Here's the drawing with two shaded views (mm, measured from the low corner). I have some questions. Coordinates: 2 decimals unless noted, no trailing zeros. Order: outer loops, then holes, each group sorted by start corner. A loop starts at its lowest first (then second) coordinate and runs counter-clockwise, first axis right, second up. Notation, with made-up numbers: (45.5, 44.5) - (64.5, 44.5) arc R26 ccw to (64.5, 66.5) - close; hole circle Ø10 at (21.25, 8.25). An arc over 180 degrees is marked (long way). Answer as a JSON object with one key per item and string values. Group by question number.
(1) Will these pins go through, and if not, where does the flat tip stop? P1, Ø1, axis at x = 5.5, z = 15, coming from the +Y side; P2, Ø5, axis at x = 4.5, z = 14.5, coming from the +Y side; P3, Ø6, axis at x = 14, z = 19.5, coming from the +Y side; P4, Ø3, axis at x = 14.5, y = 56.5, coming from the +Z side (1 decimal).
(2) Imagine slicing it at C-C, the plane z = 3. Write out the boundary of the cut face in (x, y).
(3) Please list where these lines run through material, in increasing order: probe 1 along Z at (x, y) = (10.5, 50.8); probe 2 along Y at (x, z) = (6, 13.75); probe 3 along Y at (x, z) = (10, 14.5).
(4) We'd pull the mould along Z, two halves only. Please class the marked faces 1, 2, 3 and 4: pulls with the +Z half, pulls with the -Z half, needs draft (parallel to the pull), parting line crosses it, or undercut.
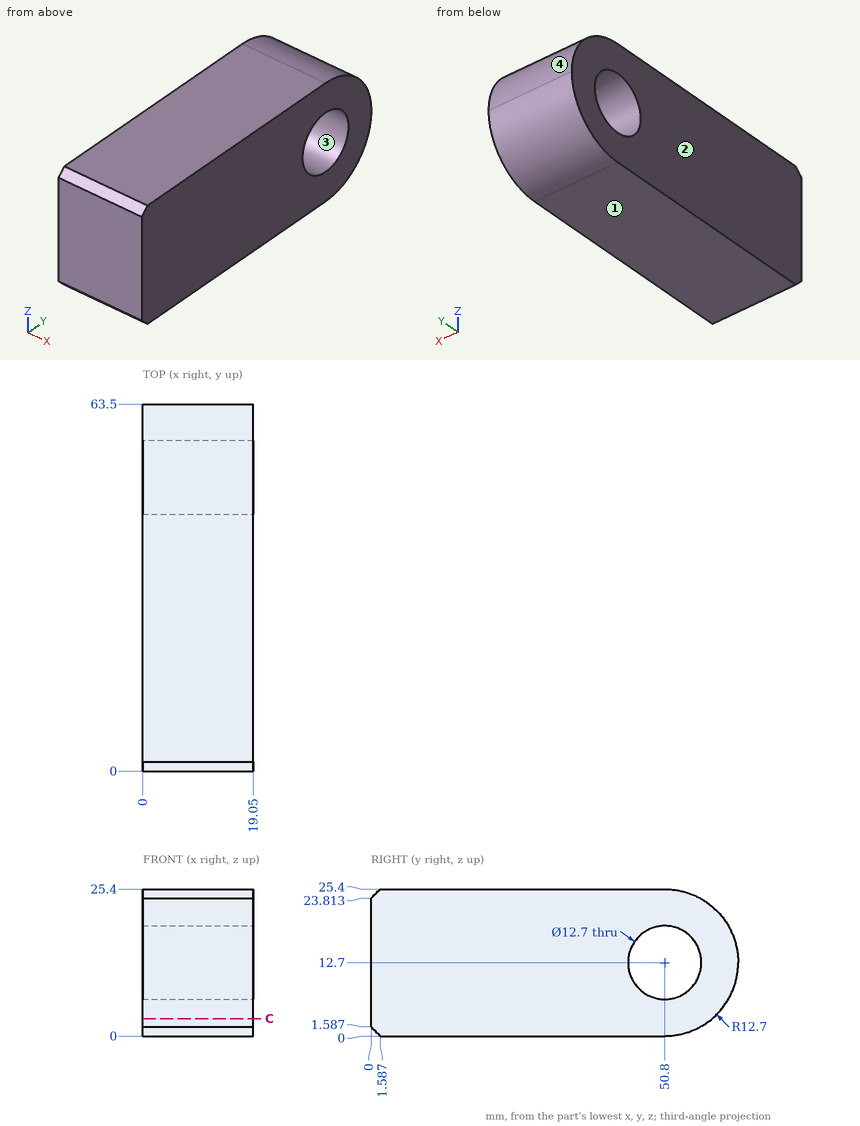
Result set:
{
 "1": {"P1": "stops at y = 63.37", "P2": "stops at y = 63.5", "P3": "stops at y = 62.92", "P4": "stops at z = 24.7"},
 "2": {"outline": "(0, 0) - (19.05, 0) - (19.05, 59) - (0, 59) - close"},
 "3": {"probe 1": "z = 0 to 6.35, 19.05 to 25.4", "probe 2": "y = 0 to 44.54, 57.06 to 63.46", "probe 3": "y = 0 to 44.71, 56.89 to 63.37"},
 "4": {"face 1": "pulls with the -Z half", "face 2": "needs draft", "face 3": "undercut", "face 4": "pulls with the +Z half"}
}
